Build history of the part. All positions in model axes, mm. Give positions to 0.01 mm unless a question says otherwise; leave off trailing zeros. Order: outer loops, then holes, each group sorted by start corner. A loop starts at its lowest first (then second) coordinate and runs counter-clockwise, first axis right, second up. Notation, with made-up numbers: M 24,7.5 L 51,7.5 A24 ccw 51,41.5 Z; hole C -24.5,49.5 d8. An arc over 180 degrees is marked long. Use CSV: the item, a comma, the result in double quotes. Start each with the question number.
Item 1: Band-saw the part on A-A on x = -7. Write the cut outline in (y, z).
Item 2: Band-saw the part on C-C on x = 24.5. Write the cut outline in (y, z).
Item 3: Wall check: line 1 along Y through (x, z) = (0, 1.85); line 2 along Y through (x, z) = (-8.5, 2.5); line 3 along Y through (x, z) = (22, 0.4). Give the ranges that are in metal, low to high.
Item 4: Pin check, flat tips, straight feed: P1, Ø2, axis at y = 13, z = 3.5, coming from the +X side; P2, Ø0.9, axis at y = 11, z = 2.5, coming from the +X side; P3, Ø1, axis at x = -25.5, z = 3.5, coming from the -Y side. Stop position of each tip, or through.
Item 5: Band-saw the part on D-D on z = 1. Give the number of separate pieces and of enclosed holes in the cut face, plus the area to 3 significant figures.
Item 6: Band-saw the part on B-B on y = 22. Write the cut outline in (x, z), plus the area to 3 significant figures.
from build123d import *

# Parameters (mm, degrees)
SKETCH1_R           = 1.5
SKETCH1_R_2         = 1.610311209
BOSS_EXTRUDE1_DEPTH = 4
CUT_EXTRUDE1_START  = -4
CUT_EXTRUDE1_DEPTH  = 4


with BuildPart() as part:
    # Sketch1 → Boss-Extrude1 (new body)
    with BuildSketch(Plane.XY):
        with BuildLine():
            Line((-40, 64.661867252), (-38.110698604, 5.904474432))
            Line((-38.110698604, 5.904474432), (-38.110698604, 1.610311209))
            Line((-38.110698604, 1.610311209), (-35.5, 2.161867252))
            Line((-35.5, 2.161867252), (-22.464466094, -10.873666654))
            Line((-22.464466094, -10.873666654), (-16.914557514, -7.843437092))
            ThreePointArc((-16.914557514, -7.843437092), (-16.338632472, -5.277165438), (-13.868441411, -6.180268964))
            Line((-13.868441411, -6.180268964), (-8.352527173, -3.168600187))
            ThreePointArc((-8.352527173, -3.168600187), (-6.823233186, -1.984189553), (-5, -1.338132748))
            Line((-5, -1.338132748), (5, -1.338132748))
            ThreePointArc((5, -1.338132748), (6.823233186, -1.984189553), (8.352527173, -3.168600187))
            Line((8.352527173, -3.168600187), (13.868441411, -6.180268964))
            ThreePointArc((13.868441411, -6.180268964), (16.338632472, -5.277165438), (16.914557514, -7.843437092))
            Line((16.914557514, -7.843437092), (22.464466094, -10.873666654))
            Line((22.464466094, -10.873666654), (35.5, 2.161867252))
            Line((35.5, 2.161867252), (38.110698604, 1.610311209))
            Line((38.110698604, 1.610311209), (38.110698604, 5.904474432))
            Line((38.110698604, 5.904474432), (40, 64.661867252))
            Line((40, 64.661867252), (40, 69.661867252))
            Line((40, 69.661867252), (-40, 69.661867252))
            Line((-40, 69.661867252), (-40, 64.661867252))
        make_face()
        with BuildLine():
            Line((16.639882489, 12.98256249), (3.11899286, 12.98256249))
            ThreePointArc((3.11899286, 12.98256249), (0, 13.661867252), (-3.11899286, 12.98256249))
            Line((-3.11899286, 12.98256249), (-15.511590599, 12.98256249))
            Line((-15.511590599, 12.98256249), (-15.511590599, 9.98256249))
            ThreePointArc((-15.511590599, 9.98256249), (-20.760848223, 9.540954041), (-25.658820737, 7.60198811))
            Line((-25.658820737, 7.60198811), (-26.230521812, 25.381927681))
            Line((-26.230521812, 25.381927681), (26.230521812, 25.381927681))
            Line((26.230521812, 25.381927681), (25.658820737, 7.60198811))
            ThreePointArc((25.658820737, 7.60198811), (21.308334072, 9.403441757), (16.639882489, 10.017875862))
            Line((16.639882489, 10.017875862), (16.639882489, 12.98256249))
        make_face(mode=Mode.SUBTRACT)
        with Locations((-34.124535685, 65.161867252)):
            Circle(SKETCH1_R, mode=Mode.SUBTRACT)
        with Locations((-14.124535685, 64.661867252)):
            Circle(SKETCH1_R, mode=Mode.SUBTRACT)
        Polygon((-26.45560174, 32.381927681), (-27.252382744, 57.161867252), (27.252382744, 57.161867252), (26.45560174, 32.381927681), align=None, mode=Mode.SUBTRACT)
        with Locations((14.124535685, 64.661867252)):
            Circle(SKETCH1_R, mode=Mode.SUBTRACT)
        with Locations((34.124535685, 65.161867252)):
            Circle(SKETCH1_R, mode=Mode.SUBTRACT)
        with Locations((-24.5, -1.838132748)):
            Circle(SKETCH1_R, mode=Mode.SUBTRACT)
        with Locations((0, 9.661867252)):
            Circle(SKETCH1_R_2, mode=Mode.SUBTRACT)
        with Locations((24.5, -1.838132748)):
            Circle(SKETCH1_R, mode=Mode.SUBTRACT)
    extrude(amount=BOSS_EXTRUDE1_DEPTH)

    # Sketch2 → Cut-Extrude1 (cut)
    with BuildSketch(Plane.XY.offset(4).offset(CUT_EXTRUDE1_START)):
        with BuildLine():
            Line((-19.116408786, -9.045639745), (-16.914557514, -7.843437092))
            ThreePointArc((-16.914557514, -7.843437092), (-16.338632472, -5.277165438), (-13.868441411, -6.180268964))
            Line((-13.868441411, -6.180268964), (-11.666590138, -4.978066311))
            ThreePointArc((-11.666590138, -4.978066311), (-17.536678859, -3.082926424), (-19.116408786, -9.045639745))
        make_face()
        with BuildLine():
            Line((16.914557514, -7.843437092), (19.116408786, -9.045639745))
            ThreePointArc((19.116408786, -9.045639745), (17.536678859, -3.082926424), (11.666590138, -4.978066311))
            Line((11.666590138, -4.978066311), (13.868441411, -6.180268964))
            ThreePointArc((13.868441411, -6.180268964), (16.338632472, -5.277165438), (16.914557514, -7.843437092))
        make_face()
    extrude(amount=CUT_EXTRUDE1_DEPTH, mode=Mode.SUBTRACT)


solid = part.part
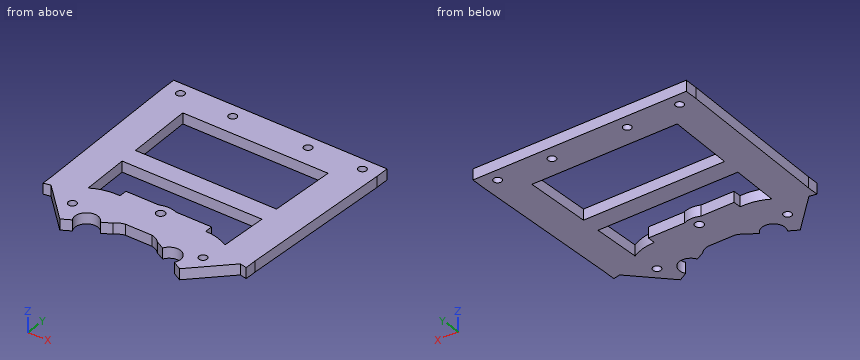
Model answer:
1,outline,"M -2.08,0 L 12.98,0 L 12.98,4 L -2.08,4 Z; M 25.38,0 L 32.38,0 L 32.38,4 L 25.38,4 Z; M 57.16,0 L 69.66,0 L 69.66,4 L 57.16,4 Z"
2,outline,"M -8.84,0 L -3.34,0 L -3.34,4 L -8.84,4 Z; M -0.34,0 L 8.22,0 L 8.22,4 L -0.34,4 Z; M 25.38,0 L 32.38,0 L 32.38,4 L 25.38,4 Z; M 57.16,0 L 69.66,0 L 69.66,4 L 57.16,4 Z"
3,line 1,"y = -1.34 to 8.05, 11.27 to 13.66, 25.38 to 32.38, 57.16 to 69.66"
3,line 2,"y = -3.25 to 12.98, 25.38 to 32.38, 57.16 to 69.66"
3,line 3,"y = -10.62 to 9.2, 25.38 to 32.38, 57.16 to 69.66"
4,P1,"stops at x = 38.37"
4,P2,"stops at x = 38.29"
4,P3,"stops at y = -8.34"
5,separate pieces,"1"
5,enclosed holes,"9"
5,area,"3,610 mm^2"
6,outline,"M -38.63,0 L -26.12,0 L -26.12,4 L -38.63,4 Z; M 26.12,0 L 38.63,0 L 38.63,4 L 26.12,4 Z"
6,area,"100 mm^2"
